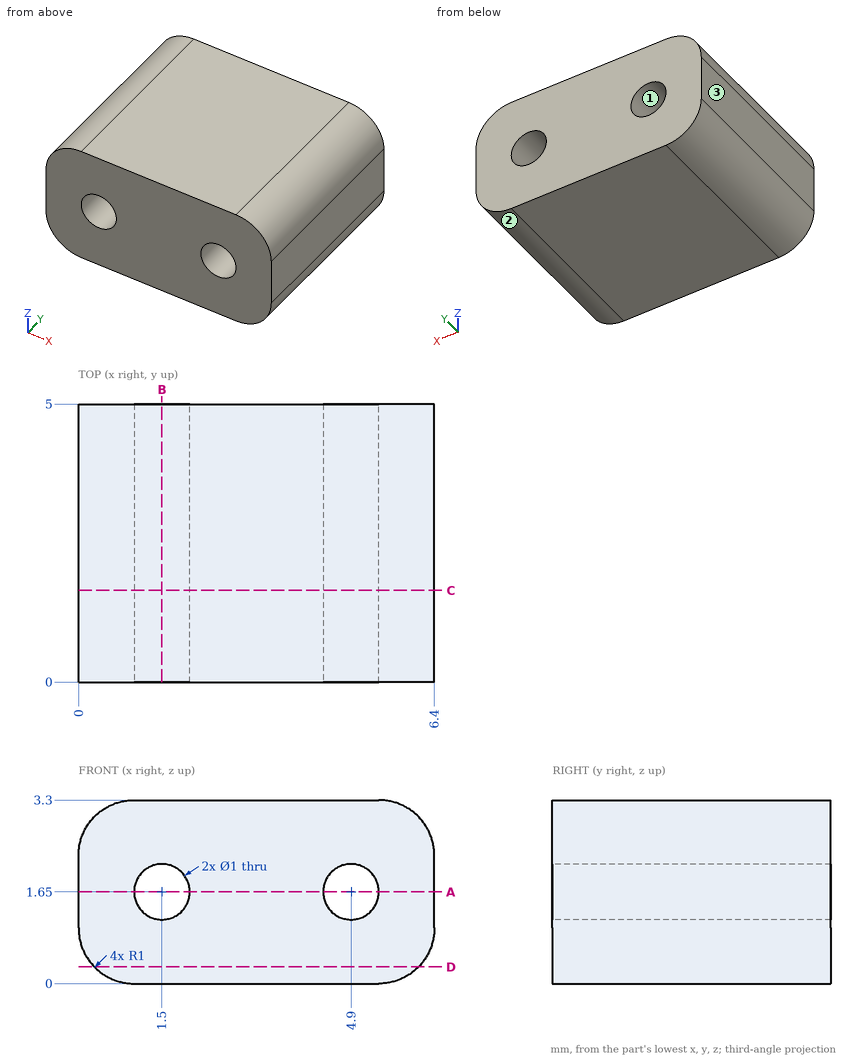
Could you check a few things on this drawing? It's one solid part, dimensions in mm from its lowest x, y, z. Coordinates: 2 decimals unless noted, no trailing zeros. Loops run counter-clockwise (first coordinate to the right, second up) from the corner with the lowest first, then second, coordinate; pieces in that order, holes last.
1. Imagine slicing it at D-D (z = 0.3). Please give me the cut outline in (x, y), and give its area (3 significant figures).
2. Imagine slicing it at C-C (y = 1.65). Please give me the cut outline in (x, z), and give its area (3 significant figures).
3. Imagine slicing it at B-B (x = 1.5). Please give me the cut outline in (y, z).
4. Imagine slicing it at A-A (z = 1.65). Please give me the cut outline in (x, y).
5. I need wall thicknesses on L1, parallel to Z at x = 1.5, y = 1.8; L2, parallel to X at y = 4.7, z = 1.95; L3, parallel to Z at x = 5.5, y = 1. Which ranges of each line are inside material? Lowest first, please.
6. We'd pull the mould along Z, two halves only. Please class the marked faces 1, 2 and 3: released by +Z, released by -Z, zero draft, split by the parting line, or undercut.
Computed values:
1. outline: (0.29, 0) - (6.11, 0) - (6.11, 5) - (0.29, 5) - close
1. area: 29.1 mm2
2. outline: (0, 1) arc R1 ccw to (1, 0) - (5.4, 0) arc R1 ccw to (6.4, 1) - (6.4, 2.3) arc R1 ccw to (5.4, 3.3) - (1, 3.3) arc R1 ccw to (0, 2.3) - close; hole circle Ø1 at (1.5, 1.65); hole circle Ø1 at (4.9, 1.65)
2. area: 18.7 mm2
3. outline: (0, 0) - (5, 0) - (5, 1.15) - (0, 1.15) - close; (0, 2.15) - (5, 2.15) - (5, 3.3) - (0, 3.3) - close
4. outline: (0, 0) - (1, 0) - (1, 5) - (0, 5) - close; (2, 0) - (4.4, 0) - (4.4, 5) - (2, 5) - close; (5.4, 0) - (6.4, 0) - (6.4, 5) - (5.4, 5) - close
5. L1: z = 0 to 1.15, 2.15 to 3.3
5. L2: x = 0 to 1.1, 1.9 to 4.5, 5.3 to 6.4
5. L3: z = 0.01 to 3.29
6. face 1: undercut
6. face 2: released by -Z
6. face 3: zero draft
